from build123d import *

# Parameters (mm, degrees)
CROQUIS1_R              = 52.5
SALIENTE_EXTRUIR1_DEPTH = 10
SALIENTE_EXTRUIR1_DRAFT = -69
CROQUIS2_R              = 78.550890647
SALIENTE_EXTRUIR2_DEPTH = 10
CROQUIS3_R              = 78.550890647
SALIENTE_EXTRUIR3_DEPTH = 10
SALIENTE_EXTRUIR3_TAPER = 69
CROQUIS4_R              = 49.5
SALIENTE_EXTRUIR4_DEPTH = 3
C_PULA1_FACE_RADIUS     = 49.5
C_PULA1_HEIGHT          = 16
CORTAR_EXTRUIR1_DEPTH   = 122.414516736
CORTAR_EXTRUIR3_REACH   = 184.352
SALIENTE_EXTRUIR5_DEPTH = 6
MATRIZL1_COUNT          = 2
MATRIZL1_PITCH          = 40


with BuildPart() as part:
    # Croquis1 → Saliente-Extruir1 (with draft: the straight prism first)
    with BuildSketch(Plane(origin=(0, 0, 0), x_dir=(1, 0, 0), z_dir=(0, 1, 0))):
        Circle(CROQUIS1_R)
    extrude(amount=SALIENTE_EXTRUIR1_DEPTH)
    # Saliente-Extruir1: the draft: its side faces are tilted about the plane it starts from
    saliente_extruir1_sides = [part.faces().sort_by_distance(p)[0] for p in [
        (-52.5, 5, 0),
    ]]
    draft(saliente_extruir1_sides, Plane(origin=(0, 0, 0), x_dir=(1, 0, 0), z_dir=(0, 1, 0)), SALIENTE_EXTRUIR1_DRAFT)

    # Croquis2 → Saliente-Extruir2 (add)
    with BuildSketch(Plane(origin=(0, 10, 0), x_dir=(1, 0, 0), z_dir=(0, 1, 0))):
        with Locations(Location((0, 0, 0), (0, 0, 270))):
            Circle(CROQUIS2_R)
    extrude(amount=SALIENTE_EXTRUIR2_DEPTH)

    # Croquis3 → Saliente-Extruir3 (add)
    with BuildSketch(Plane(origin=(0, 20, 0), x_dir=(1, 0, 0), z_dir=(0, 1, 0))):
        with Locations(Location((0, 0, 0), (0, 0, 270))):
            Circle(CROQUIS3_R)
    extrude(amount=SALIENTE_EXTRUIR3_DEPTH, taper=SALIENTE_EXTRUIR3_TAPER)

    # Croquis4 → Saliente-Extruir4 (add)
    with BuildSketch(Plane(origin=(0, 30, 0), x_dir=(1, 0, 0), z_dir=(0, 1, 0))):
        with Locations(Location((0, 0, 0), (0, 0, 270))):
            Circle(CROQUIS4_R)
    extrude(amount=SALIENTE_EXTRUIR4_DEPTH)

    # Cúpula1: a dome of height H over a round flat face of radius A is a cap of a sphere of radius (A * A + H * H) / (2 * H)
    c_pula1_r = (C_PULA1_FACE_RADIUS * C_PULA1_FACE_RADIUS + C_PULA1_HEIGHT * C_PULA1_HEIGHT) / (2 * C_PULA1_HEIGHT)
    c_pula1_base = Plane((0, 33, 0), z_dir=(0, 1, 0))
    with Locations(c_pula1_base.offset(C_PULA1_HEIGHT - c_pula1_r)):
        c_pula1_ball = Sphere(c_pula1_r, mode=Mode.PRIVATE)
    add(split(c_pula1_ball, bisect_by=c_pula1_base, keep=Keep.TOP, mode=Mode.PRIVATE))

    # Croquis6 → Cortar-Extruir1 (cut, through all)
    with BuildSketch(Plane(origin=(0, 0, 0), x_dir=(0, 0, -1), z_dir=(1, 0, 0))):
        Polygon((-49.5, 33), (55.064393683, 0.984378507), (52.5, 0), (-52.5, 0), (-78.550890647, 10), (-78.550890647, 20), align=None)
    extrude(amount=CORTAR_EXTRUIR1_DEPTH, mode=Mode.SUBTRACT)

    # Cortar-Extruir3: up to this plane
    cortar_extruir3_end = Plane(origin=(78.550890647, 33, 49.5), z_dir=(0, -0.9561843075173418, 0.2927653839810668))
    # Croquis9 → Cortar-Extruir3 (cut, up to the surface)
    with BuildSketch(Plane.XY.offset(78.550890647), mode=Mode.PRIVATE) as cortar_extruir3_sk1:
        Polygon((0, 0), (-21.79627584, 30), (0, 30), align=None)
    cortar_extruir3_tool1 = split(extrude(cortar_extruir3_sk1.sketch, amount=-CORTAR_EXTRUIR3_REACH, mode=Mode.PRIVATE), bisect_by=cortar_extruir3_end, keep=Keep.BOTH, mode=Mode.PRIVATE)
    add(cortar_extruir3_tool1.solids().sort_by_distance((-7.265425, 20, 78.550891))[0], mode=Mode.SUBTRACT)

    # Croquis11 → Saliente-Extruir5 (add)
    with BuildSketch(Plane.XY.offset(20)):
        Polygon((-63.346461172, 16.251599406), (-52.5, 0), (-41.36, 0), (-59.921256857, -15.574743783), (-77.919309928, 5.874500625), align=None)
    saliente_extruir5 = extrude(amount=SALIENTE_EXTRUIR5_DEPTH)

    # MatrizL1: Saliente-Extruir5 ×2
    with Locations(*[(0, 0, -i * MATRIZL1_PITCH) for i in range(1, MATRIZL1_COUNT)]):
        add(saliente_extruir5)


solid = part.part
Input: part model. Units: mm. Frame: model coordinates. A direction names the side the tool comes from. Coordinates: 2 decimals unless noted, no trailing zeros. Loops run counter-clockwise (first coordinate to the right, second up) from the corner with the lowest first, then second, coordinate; pieces in that order, holes last. Notation, with made-up numbers: (-16.75, 60.25) -> (31.25, 60.25) arc R18 ccw to (31.25, 73.25) -> close; hole circle Ø11 at (57.25, 13). An arc over 180 degrees is marked (long way). Write each question's results on one line, items separated by ' | '. Start each with the question number.
Q1. Section A-A, the plane z = 0. Return the cut outline in (x, y), plus the area to 3 significant figures.
Q2. Section B-B, the plane y = 15. Return the cut outline in (x, z), plus the area to 3 significant figures.
Q3. Ray query, line 1 (Y direction, x = -40.5, z = 46); line 2 (X direction, y = 17.5, z = -34); line 3 (Y direction, x = -10, z = 26.5). Return the intervals inside material, ascending. Write a range as from..to.
Q4. Reachability of faces 4 (the cylindrical face through (2.18, 31.48, -49.45)), 5 (the flat face through (-59, -3, 26)), 6 (the flat face through (-59, -3, 20)), 7 (the flat face through (-50.51, -7.68, -17.04)) from +Z, -Z, +X, -X, +Y, -Y: full face, straight path, thin tool, end or side. Return the list, or none.
Q5. Pull-direction query (Y, two-part tool) for faces 1 (the flat face through (-51, 0, -17)), 2 (the flat face through (-59, -3, -20)), 3 (the conical face through (-12.043, 29.514, -52.399)); classes: released by +Y, released by -Y, zero draft, split by the parting line, or undercut.
Q6. Pin query (flat end, axial travel): pin 1 (7.5 mm diameter, centred on x = -66.5, y = -7.5, fed in from -Z); pin 2 (12 mm diameter, centred on x = 20, z = -38.5, fed in from +Y); pin 3 (3 mm diameter, centred on x = -51, z = -18, fed in from +Y). Return the tip coordinate at first contact, or that it passes through.
Found:
1) outline: (-78.55, 10) -> (-52.5, 0) -> (0, 0) -> (-12.96, 17.84) -> (78.55, 17.84) -> (78.55, 20) -> (52.5, 30) -> (49.5, 30) -> (49.5, 33) arc R84.57 ccw to (-49.5, 33) -> (-49.5, 30) -> (-52.5, 30) -> (-78.55, 20) -> close | area: 4,180 mm2
2) outline: (-10.9, -9.29) -> (-10.9, 77.79) arc R78.55 ccw (long way) to (78, -9.29) -> close | area: 12,900 mm2
3) line 1: 3.37..26.63 | line 2: -70.81..70.81 | line 3: 0..13.76, 25.96..44.12
4) face 4: +Y | face 5: +Z, -X, -Y | face 6: -X, -Y | face 7: +Z, -Z, +X, -Y
5) face 1: undercut | face 2: zero draft | face 3: released by +Y
6) pin 1: z = -20 | pin 2: y = 40.29 | pin 3: y = 29.97
